Autodesk Inventor part; units mm, degrees
ref_plane "YZ Plane" through (0, 0, 0) normal (1, 0, 0) x (0, 1, 0)
ref_plane "XZ Plane" through (0, 0, 0) normal (0, 1, 0) x (-1, 0, 0)
ref_plane "XY Plane" through (0, 0, 0) normal (0, 0, 1) x (1, 0, 0)
sketch "Sketch1" plane through (0, 0, 0) normal (0, 0, 1) x (1, 0, 0)
  circle A0 centre (0, 0) radius 40
  line L0 (0, 0) -> (32.5, 0)
  line L1 (0, 0) -> (0, 32.5)
  circle A1 centre (0, 32.5) radius 3
  circle A2 centre (32.5, 0) radius 3
  circle A3 centre (0, -32.5) radius 3
  circle A4 centre (-32.5, 0) radius 3
  circle A5 centre (0, 0) radius 4
  dimension "d0" = 80
  dimension "d1" = 32.5
  dimension "d2" = 32.5
  dimension "d3" = 6
  dimension "d4" = 6
  dimension "d5" = 8
extrude "Extrusion1" add sketch "Sketch1" along normal blind 2
sketch "Sketch2" plane through (0, 0, 0) normal (0, 0, -1) x (-1, 0, 0)
  circle A0 centre (0, 0) radius 4
  circle A1 centre (0, 0) radius 15
  dimension "d8" = 30
extrude "Extrusion2" add sketch "Sketch2" along normal blind 20
sketch "Sketch3" plane through (0, 0, -20) normal (0, 0, -1) x (-1, 0, 0)
  circle A0 centre (0, 0) radius 15
  line L0 (-10.7651, -10.4457) -> (-10.7651, 10.4457)
  circle A1 centre (0, 0) radius 15
extrude "Extrusion3" cut sketch "Sketch3" against normal blind 20 contours L0 A0 picked at (-11.4387, 2.6145)
sketch "Sketch4" plane through (10.7651, -10.4457, -20) normal (1, 0, 0) x (0, 0, -1)
  circle A0 centre (-11, 10.4457) radius 2.95
  point P0 (-20, 10.4457)
  dimension "d13" = 5.9
extrude "Extrusion4" cut sketch "Sketch4" against normal blind 11.75
thread "Thread1"
properties part number "Sprocket Adapter"
Read the model definition and answer for the solid it produces. Units are mm, in the model's axes. A direction names the side the tool comes from. Coordinates: 2 decimals unless noted, no trailing zeros. Order: outer loops, then holes, each group sorted by start corner. A loop starts at its lowest first (then second) coordinate and runs counter-clockwise, first axis right, second up. Notation, with made-up numbers: (43.25, 31) - (101.25, 31) arc R17 cw to (101.25, 47) - close; hole circle Ø10 at (37.5, 62). An arc over 180 degrees is marked (long way). Answer as a JSON object with one key per item and string values. Group by question number.
Item 1: Consider probe 1 along Y at (x, z) = (0, 0.55); probe 2 along Z at (x, y) = (4.5, 0); probe 3 along Z at (x, y) = (24.5, 25). Determine where each line is inside the solid, lowest interval first. Write a range as from..to.
Item 2: A tool of negligible diameter and unlimited length cuts with its end or side. For faces 4 (the face through (17, 1, 0)), 5 (the face through (10.765, -0.1, -12.4)), 6 (the face through (-35.5, -0.1, 1)), from which of +Z, -Z, +X, -X, +Y, -Y can it reach the whole face along a straight path? Write none if from no direction.
Item 3: Flat-ended cylindrical pins translate along their axes: P1, Ø8, axis at x = -23, y = -1.5, coming from the -Z side; P2, Ø6, axis at x = -1.5, z = -2, coming from the -Y side; P3, Ø1, axis at x = 4.5, z = -17.5, coming from the -Y side. Find the tip coordinate at first contact, or state that the pin passes through.
Item 4: Section A-A (x = 32.5) is taken. Give the vertices of the cut face in (y, z).
Item 5: The mould has two halves that part along X. Classify faces 1 (the face through (-2.21, -34.53, 0.99)), 2 (the face through (-15, 0, -10)), 3 (the face through (6.789, 0.886, -11.814)): +X half, -X half, draft (parallel to the pull), parting line (faces both ways), or undercut.
Item 6: Section C-C (z = -9) is taken. Give the vertices of the cut face in (x, y), plus the area to 3 significant figures.
Item 7: Section D-D (y = -14) is taken. Give the vertices of the cut face in (x, z).
Results are:
{
 "1": {"probe 1": "y = -40..-35.5, -29.5..-4, 4..29.5, 35.5..40", "probe 2": "z = -20..-11.95, -6.05..2", "probe 3": "z = 0..2"},
 "2": {"face 4": "-Z", "face 5": "-Z, +X, +Y, -Y", "face 6": "+Z, -Z"},
 "3": {"P1": "stops at z = 0", "P2": "stops at y = -40", "P3": "stops at y = -14.46"},
 "4": {"outline": "(-23.32, 0) - (-3, 0) - (-3, 2) - (-23.32, 2) - close; (3, 0) - (23.32, 0) - (23.32, 2) - (3, 2) - close"},
 "5": {"face 1": "undercut", "face 2": "parting line", "face 3": "draft"},
 "6": {"outline": "(2.7, -2.95) arc R4 cw (long way) to (2.7, 2.95) - (10.77, 2.95) - (10.77, 10.45) arc R15 ccw (long way) to (10.77, -10.45) - (10.77, -2.95) - close", "area": "553 mm^2"},
 "7": {"outline": "(-37.47, 0) - (-5.39, 0) - (-5.39, -20) - (5.39, -20) - (5.39, 0) - (37.47, 0) - (37.47, 2) - (-37.47, 2) - close"}
}
